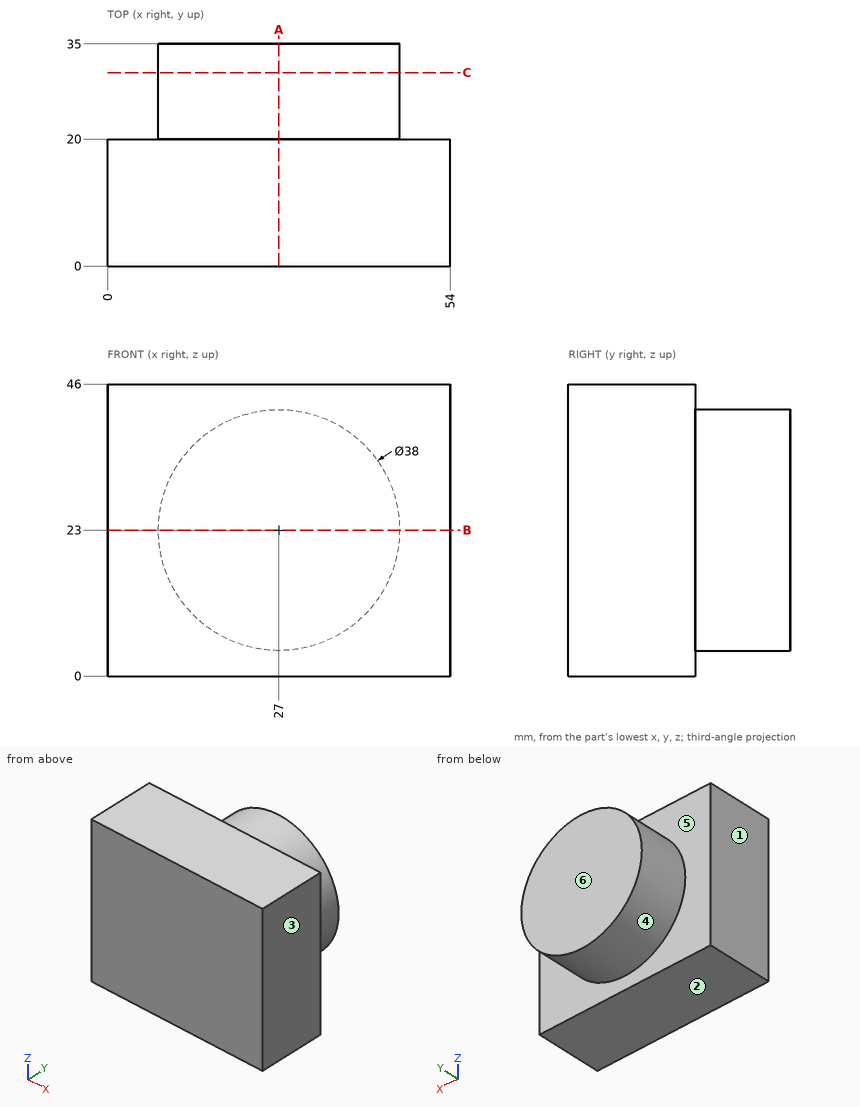
Can you work these out from the drawing? Everything is in mm from the part's minimum corner. A direction names the side the tool comes from. Give positions to 0.01 mm unless a question says otherwise; leave off trailing zeros. Order: outer loops, then holes, each group sorted by start corner. A loop starts at its lowest first (then second) coordinate and runs counter-clockwise, first axis right, second up.
1. I need wall thicknesses on L1, parallel to Y at x = 43, z = 42; L2, parallel to X at y = 29.5, z = 7; L3, parallel to X at y = 25, z = 27. Which ranges of each line are inside material? Lowest first, please.
2. Suppose I cut it at C-C (y = 30.5). List the corners of the cut face in (x, z) for me.
3. Suppose I cut it at B-B (z = 23). List the corners of the cut face in (x, y) for me.
4. For the marked faces 5 and 6, which set-ups out of +Z, -Z, +X, -X, +Y, -Y let a thin tool reach every point of the face, with its end or its side?
5. Suppose I cut it at A-A (x = 27). List the corners of the cut face in (y, z) for me, plus the area to 3 significant figures.
6. We'd pull the mould along X, two halves only. Please class the marked faces 1, 2, 3 and 4: pulls with the +X half, pulls with the -X half, needs draft (parallel to the pull), parting line crosses it, or undercut.
Solved:
1. L1: y = 0 to 20
1. L2: x = 16.75 to 37.25
1. L3: x = 8.43 to 45.57
2. outline: circle Ø38 at (27, 23)
3. outline: (0, 0) - (54, 0) - (54, 20) - (46, 20) - (46, 35) - (8, 35) - (8, 20) - (0, 20) - close
4. face 5: +Y
4. face 6: +Z, -Z, +X, -X, +Y
5. outline: (0, 0) - (20, 0) - (20, 4) - (35, 4) - (35, 42) - (20, 42) - (20, 46) - (0, 46) - close
5. area: 1,490 mm2
6. face 1: pulls with the -X half
6. face 2: needs draft
6. face 3: pulls with the +X half
6. face 4: parting line crosses it
